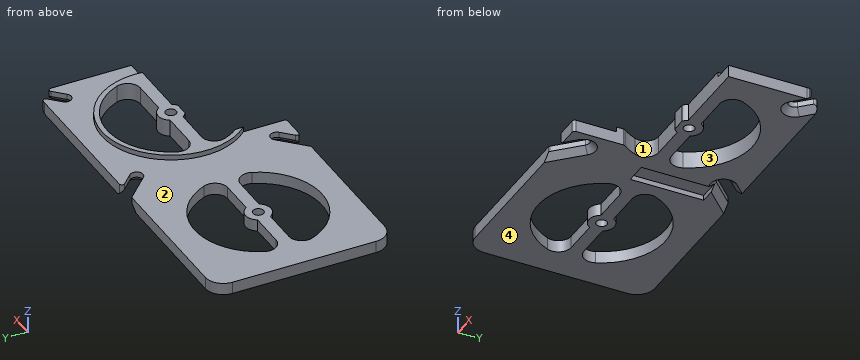
Autodesk Inventor part; units mm, degrees
ref_plane "YZ Plane" through (0, 0, 0) normal (1, 0, 0) x (0, 1, 0)
ref_plane "XZ Plane" through (0, 0, 0) normal (0, 1, 0) x (-1, 0, 0)
ref_plane "XY Plane" through (0, 0, 0) normal (0, 0, 1) x (1, 0, 0)
sketch "Sketch1" plane through (0, 0, 0) normal (0, 0, 1) x (1, 0, 0)
  line L0 (-95.2, -35.2) -> (28.2, -35.2)
  line L1 (35.2, -28.2) -> (35.2, 28.2)
  line L2 (28.2, 35.2) -> (-95.2, 35.2)
  line L3 (-102.2, 28.2) -> (-102.2, -28.2)
  arc A0 (-95.2, 35.2) -> (-102.2, 28.2) centre (-95.2, 28.2) ccw
  arc A1 (35.2, 28.2) -> (28.2, 35.2) centre (28.2, 28.2) ccw
  arc A2 (-102.2, -28.2) -> (-95.2, -35.2) centre (-95.2, -28.2) ccw
  arc A3 (28.2, -35.2) -> (35.2, -28.2) centre (28.2, -28.2) ccw
  line L4 (24.8747, -2.5) -> (24.8747, 2.5) construction
  line L5 (-24.8747, 2.5) -> (-24.8747, -2.5) construction
  line L6 (24.8747, -2.5) -> (-24.8747, 2.5) construction
  line L7 (24.8747, 2.5) -> (-24.8747, -2.5) construction
  arc A4 (-23.1756, -9.375) -> (23.1756, -9.375) centre (0, 0) ccw
  arc A5 (23.1756, 9.375) -> (-23.1756, 9.375) centre (0, 0) ccw
  arc A6 (-18.5405, -2.5) -> (-23.1756, -9.375) centre (-18.5405, -7.5) ccw
  arc A7 (-23.1756, 9.375) -> (-18.5405, 2.5) centre (-18.5405, 7.5) ccw
  arc A8 (23.1756, -9.375) -> (18.5405, -2.5) centre (18.5405, -7.5) ccw
  arc A9 (18.5405, 2.5) -> (23.1756, 9.375) centre (18.5405, 7.5) ccw
  line L8 (-4.3301, 2.5) -> (-18.5405, 2.5)
  line L9 (-18.5405, -2.5) -> (-4.3301, -2.5)
  line L10 (4.3301, -2.5) -> (18.5405, -2.5)
  line L11 (18.5405, 2.5) -> (4.3301, 2.5)
  arc A10 (-4.3301, -2.5) -> (4.3301, -2.5) centre (0, 0) ccw
  arc A11 (4.3301, 2.5) -> (-4.3301, 2.5) centre (0, 0) ccw
  line L12 (-18.5405, 7.5) -> (18.5405, 7.5) construction
  line L13 (18.5405, -7.5) -> (-18.5405, -7.5) construction
  line L14 (0, 0) -> (0, -35.2) construction
  line L15 (0, 0) -> (0, 35.2) construction
  line L16 (0, 0) -> (35.2, 0) construction
  line L17 (-33.5, -35.2) -> (-33.5, 35.2) construction
  arc A12 (-90.1756, -9.375) -> (-43.8244, -9.375) centre (-67, 0) ccw
  arc A13 (-43.8244, 9.375) -> (-90.1756, 9.375) centre (-67, 0) ccw
  arc A14 (-43.8244, -9.375) -> (-48.4595, -2.5) centre (-48.4595, -7.5) ccw
  arc A15 (-48.4595, 2.5) -> (-43.8244, 9.375) centre (-48.4595, 7.5) ccw
  arc A16 (-85.5405, -2.5) -> (-90.1756, -9.375) centre (-85.5405, -7.5) ccw
  arc A17 (-90.1756, 9.375) -> (-85.5405, 2.5) centre (-85.5405, 7.5) ccw
  line L18 (-62.6699, 2.5) -> (-48.4595, 2.5)
  line L19 (-48.4595, -2.5) -> (-62.6699, -2.5)
  line L20 (-71.3301, -2.5) -> (-85.5405, -2.5)
  line L21 (-85.5405, 2.5) -> (-71.3301, 2.5)
  arc A18 (-71.3301, -2.5) -> (-62.6699, -2.5) centre (-67, 0) ccw
  arc A19 (-62.6699, 2.5) -> (-71.3301, 2.5) centre (-67, 0) ccw
  point P0 (0, 0)
  point P1 (0, 0)
  dimension "d63" = 67
  dimension "d1" = 7
  dimension "d3" = 5
  dimension "d4" = 25
  dimension "d5" = 5
  dimension "d7" = 5
  dimension "d59" = 70.4
  dimension "d60" = 137.4
extrude "Extrusion1" add sketch "Sketch1" along normal blind 4.7
sketch "Sketch2" plane through (0, 0, 4.7) normal (0, 0, 1) x (1, 0, 0)
  circle A0 centre (0, 0) radius 27
  arc A1 (23.1756, 9.375) -> (-23.1756, 9.375) centre (0, 0) ccw
  arc A2 (18.5405, 2.5) -> (23.1756, 9.375) centre (18.5405, 7.5) ccw
  line L0 (18.5405, 2.5) -> (4.3301, 2.5)
  arc A3 (4.3301, 2.5) -> (-4.3301, 2.5) centre (0, 0) ccw
  line L1 (-4.3301, 2.5) -> (-18.5405, 2.5)
  arc A4 (-23.1756, 9.375) -> (-18.5405, 2.5) centre (-18.5405, 7.5) ccw
  line L2 (-18.5405, -2.5) -> (-4.3301, -2.5)
  arc A5 (-4.3301, -2.5) -> (4.3301, -2.5) centre (0, 0) ccw
  line L3 (4.3301, -2.5) -> (18.5405, -2.5)
  arc A6 (23.1756, -9.375) -> (18.5405, -2.5) centre (18.5405, -7.5) ccw
  arc A7 (-23.1756, -9.375) -> (23.1756, -9.375) centre (0, 0) ccw
  arc A8 (-18.5405, -2.5) -> (-23.1756, -9.375) centre (-18.5405, -7.5) ccw
  line L4 (28.2, 35.2) -> (-95.2, 35.2)
  arc A9 (-95.2, 35.2) -> (-102.2, 28.2) centre (-95.2, 28.2) ccw
  line L5 (-102.2, 28.2) -> (-102.2, -28.2)
  arc A10 (-102.2, -28.2) -> (-95.2, -35.2) centre (-95.2, -28.2) ccw
  line L6 (-95.2, -35.2) -> (28.2, -35.2)
  arc A11 (28.2, -35.2) -> (35.2, -28.2) centre (28.2, -28.2) ccw
  line L7 (35.2, -28.2) -> (35.2, 28.2)
  arc A12 (35.2, 28.2) -> (28.2, 35.2) centre (28.2, 28.2) ccw
  dimension "d10" = 54
extrude "Extrusion2" add sketch "Sketch2" along normal blind 2 contours A0
sketch "Sketch3" plane through (0, 0, 0) normal (0, 0, -1) x (-1, 0, 0)
  line L0 (-27.5, -27.5) -> (27.5, -27.5) construction
  line L1 (27.5, -27.5) -> (27.5, 27.5) construction
  line L2 (27.5, 27.5) -> (-27.5, 27.5) construction
  line L3 (-27.5, 27.5) -> (-27.5, -27.5) construction
  line L4 (-27.5, -27.5) -> (27.5, 27.5) construction
  line L5 (27.5, -27.5) -> (-27.5, 27.5) construction
  line L6 (-27.5, 27.5) -> (-36.9678, 36.9678) construction
  line L7 (-25.7322, 29.2678) -> (-35.2, 38.7355)
  line L8 (-38.7355, 35.2) -> (-29.2678, 25.7322)
  arc A0 (-29.2678, 25.7322) -> (-25.7322, 29.2678) centre (-27.5, 27.5) ccw
  arc A1 (-35.2, 38.7355) -> (-38.7355, 35.2) centre (-36.9678, 36.9678) ccw
  line L9 (95.2, 35.2) -> (-28.2, 35.2) construction
  arc A2 (-38.7355, -35.2) -> (-35.2, -38.7355) centre (-36.9678, -36.9678) ccw
  line L10 (-29.2678, -25.7322) -> (-38.7355, -35.2)
  line L11 (-35.2, -38.7355) -> (-25.7322, -29.2678)
  arc A3 (-25.7322, -29.2678) -> (-29.2678, -25.7322) centre (-27.5, -27.5) ccw
  arc A4 (35.2, -38.7355) -> (38.7355, -35.2) centre (36.9678, -36.9678) ccw
  line L12 (25.7322, -29.2678) -> (35.2, -38.7355)
  line L13 (38.7355, -35.2) -> (29.2678, -25.7322)
  arc A5 (29.2678, -25.7322) -> (25.7322, -29.2678) centre (27.5, -27.5) ccw
  arc A6 (38.7355, 35.2) -> (35.2, 38.7355) centre (36.9678, 36.9678) ccw
  line L14 (29.2678, 25.7322) -> (38.7355, 35.2)
  line L15 (35.2, 38.7355) -> (25.7322, 29.2678)
  arc A7 (25.7322, 29.2678) -> (29.2678, 25.7322) centre (27.5, 27.5) ccw
  arc A8 (62.6699, -2.5) -> (71.3301, -2.5) centre (67, 0) ccw construction
  line L16 (67, 0) -> (0, 0) construction
  line L17 (134, 0) -> (67, 0) construction
  arc A9 (92.7322, 29.2678) -> (96.2678, 25.7322) centre (94.5, 27.5) ccw
  line L18 (96.2678, 25.7322) -> (105.7355, 35.2)
  arc A10 (105.7355, 35.2) -> (102.2, 38.7355) centre (103.9678, 36.9678) ccw
  line L19 (102.2, 38.7355) -> (92.7322, 29.2678)
  line L20 (28.2645, 35.2) -> (37.7322, 25.7322)
  arc A11 (37.7322, 25.7322) -> (41.2678, 29.2678) centre (39.5, 27.5) ccw
  line L21 (41.2678, 29.2678) -> (31.8, 38.7355)
  arc A12 (31.8, 38.7355) -> (28.2645, 35.2) centre (30.0322, 36.9678) ccw
  line L22 (31.8, -38.7355) -> (41.2678, -29.2678)
  arc A13 (41.2678, -29.2678) -> (37.7322, -25.7322) centre (39.5, -27.5) ccw
  line L23 (37.7322, -25.7322) -> (28.2645, -35.2)
  arc A14 (28.2645, -35.2) -> (31.8, -38.7355) centre (30.0322, -36.9678) ccw
  line L24 (105.7355, -35.2) -> (96.2678, -25.7322)
  arc A15 (96.2678, -25.7322) -> (92.7322, -29.2678) centre (94.5, -27.5) ccw
  line L25 (92.7322, -29.2678) -> (102.2, -38.7355)
  arc A16 (102.2, -38.7355) -> (105.7355, -35.2) centre (103.9678, -36.9678) ccw
  point P0 (-32.2339, 32.2339)
  point P1 (129.6699, -2.5)
  point P2 (138.3301, -2.5)
  dimension "d68" = 55
  dimension "d70" = 5
  dimension "d73" = 360
  dimension "d211" = 67
  dimension "d214" = 67
  dimension "d221" = 360
extrude "Extrusion3" cut sketch "Sketch3" against normal through all contours A0 L8 A1 L7 | L10 A3 L11 A2 | L12 L22 L13 A4 | L12 L23 L13 L22 | L12 A5 L13 L23 | L14 L21 L15 A6 | L14 L20 L15 L21 | L14 A7 L15 L20
chamfer "Chamfer1" distance 2.5 angle 45 12 edges at (28.3939, 31.9294, 0) (25.7322, 25.7322, 0) (31.9294, 28.3939, 0) (-28.6983, 32.2339, 0) (-25.7322, 25.7322, 0) (-34.0017, 30.4661, 0) (-25.7322, -25.7322, 0) (-34.0017, -30.4661, 0) (-28.6983, -32.2339, 0) (25.7322, -25.7322, 0) (28.3939, -31.9294, 0) (31.9294, -28.3939, 0)
fillet "Fillet1" radius 1 8 edges at (34.5911, -31.0555, 3.6) (31.0555, -34.5911, 3.6) (31.0555, 34.5911, 3.6) (34.5911, 31.0555, 3.6) (-31.6645, 35.2, 3.6) (-38.7355, 35.2, 3.6) (-31.6645, -35.2, 3.6) (-38.7355, -35.2, 3.6)
sketch "Sketch7" plane through (0, 0, 0) normal (0, 0, -1) x (-1, 0, 0)
  arc A0 (-4.3301, -2.5) -> (4.3301, -2.5) centre (0, 0) ccw construction
  arc A1 (62.6699, -2.5) -> (71.3301, -2.5) centre (67, 0) ccw
  point P0 (0, 0)
hole "Hole2" at (0, 0, 0) at (-67, 0, 0) direction (0, 0, 1) diameter 4.2 end through all
sketch "Sketch4" plane through (0, 0, 0) normal (0, 0, -1) x (-1, 0, 0)
  line L0 (19.8, -4.2) -> (19.8, -35.2)
  line L1 (19.8, -35.2) -> (-35.2, -35.2)
  line L2 (-35.2, -35.2) -> (-35.2, -4.2)
  line L3 (19.8, -4.2) -> (-35.2, -4.2)
  line L4 (102.2, -35.2) -> (-35.2, -35.2) construction
  line L5 (-35.2, -35.2) -> (-35.2, 35.2) construction
  line L6 (-35.2, 35.2) -> (102.2, 35.2) construction
  line L7 (102.2, 35.2) -> (102.2, -35.2) construction
  line L8 (28.1289, 35.2) -> (42.2711, 35.2) construction
  line L9 (-35.2, 28.1289) -> (-35.2, -28.1289) construction
  line L10 (-28.2, -35.2) -> (28.1289, -35.2) construction
  line L11 (102.2, -28.2) -> (102.2, 28.2) construction
  line L12 (-4.3301, -2.5) -> (-18.5405, -2.5)
  line L13 (-4.3301, -2.5) -> (-35.2, -2.5)
  line L14 (-35.2, -2.5) -> (-35.2, -4.2)
  line L15 (-35.2, -4.2) -> (-4.3301, -4.2)
  line L16 (-4.3301, -4.2) -> (-4.3301, -2.5)
  point P0 (-28.1289, 35.2)
  point P1 (-28.1289, -35.2)
  dimension "d39" = 31
  dimension "d41" = 55
extrude "Extrusion4" cut sketch "Sketch4" against normal through all
fillet "Fillet2" radius 1 2 edges at (-19.8, -15.263, 3.35) (-19.8, -35.2, 2.35)
sketch "Sketch8" plane through (0, 0, 0) normal (0, 0, -1) x (-1, 0, 0)
  line L0 (0, 0) -> (35.5, 0) construction
  line L1 (35.5, 0) -> (71, 0) construction
  line L2 (32.5, 32.5) -> (32.5, -32.5) construction
  line L3 (32.5, -32.5) -> (-32.5, -32.5) construction
  line L4 (-32.5, -32.5) -> (-32.5, 32.5) construction
  line L5 (-32.5, 32.5) -> (32.5, 32.5) construction
  line L6 (99.5, 32.5) -> (99.5, -32.5) construction
  line L7 (99.5, -32.5) -> (34.5, -32.5) construction
  line L8 (34.5, -32.5) -> (34.5, 32.5) construction
  line L9 (34.5, 32.5) -> (99.5, 32.5) construction
  line L10 (96.3694, 32.5) -> (96.3694, 35.2) construction
  line L11 (99.5, 26.6962) -> (102.2, 26.6962) construction
  line L12 (92.7868, -32.5) -> (92.7868, -35.2) construction
  line L13 (102.2, -28.2) -> (102.2, 28.2) construction
  line L14 (42.2711, -35.2) -> (95.2, -35.2) construction
  line L15 (-35.2, -1.5) -> (-35.2, 28.2) construction
  line L16 (-35.2, 21.6184) -> (-32.5, 21.6184) construction
  line L17 (95.2, 35.2) -> (42.2711, 35.2) construction
  line L18 (29.4901, 25.1562) -> (37.9558, 25.1562)
  line L19 (37.9558, 25.1562) -> (37.9558, -3.6366)
  line L20 (37.9558, -3.6366) -> (29.4901, -3.6366)
  line L21 (29.4901, -3.6366) -> (29.4901, 25.1562)
  dimension "d131" = 65
extrude "Extrusion6" cut sketch "Sketch8" against normal blind 2
equation "\"Offset\" = 0.3"
equation "\"d56\" = 0.3"
properties part number "V4 in walldual"
CAD build for the part. Positions are in the model's coordinates, mm. Face numbers are marked on the shaded views. A direction names the side the tool comes from. Coordinates: 2 decimals unless noted, no trailing zeros. Order: outer loops, then holes, each group sorted by start corner. A loop starts at its lowest first (then second) coordinate and runs counter-clockwise, first axis right, second up. Notation, with made-up numbers: M 25.5,67.5 L 66.5,67.5 A18 cw 66.5,93.5 Z; hole C 73,-21 d11. An arc over 180 degrees is marked long. Answer as CSV lines item,"result".
1) Cut at B-B (y = -11). List the corners of the cut face in (x, z).
Verdict:
outline,"M -102.2,0 L -89.45,0 L -89.45,4.7 L -102.2,4.7 Z; M -44.55,0 L -22.45,0 L -22.45,6.7 L -24.66,6.7 L -24.66,4.7 L -44.55,4.7 Z"
2) Drill centre lines: L1, parallel to X at y = 0, z = 3.6; L2, parallel to Y at x = -61, z = 4.25; L3, parallel to Y at x = -51, z = 3.25. Where is each one in solid material? Low to high. Write a range as from..to.
Verdict:
L1,"-102.2..-69.1, -64.9..-2.1, 2.1..35.2"
L2,"-35.2..-24.27, -2.5..2.5, 24.27..35.2"
L3,"-35.2..-19.21, -2.5..2.5, 19.21..35.2"
3) 3-axis set-ups, long thin cutter, end or side, ignore diameter. For the marked faces 3 and 4: which of +Z, -Z, +X, -X, +Y, -Y reach the whole face in a straight line?
Verdict:
face 3,"+Z, -Z"
face 4,"-Z, +X, -X, +Y, -Y"
4) Mould opens along X. For the marked faces 1 and 2 say: released by +X, released by -X, zero draft, split by the parting line, or undercut.
Verdict:
face 1,"undercut"
face 2,"zero draft"
5) Flat gauge pins, fed straight in: P1, Ø5, axis at x = -67, y = 0, coming from the +Z side; P2, Ø3.5, axis at x = 14, z = 2.5, coming from the -Y side; P3, Ø1.5, axis at y = -23, z = 4, coming from the +X side. Where does each tip first touch, or does it go through?
Verdict:
P1,"z = 4.7"
P2,"y = -2.5"
P3,"x = -19.8"
6) Cut at A-A (x = -67). List the corners of the cut face in (y, z), then the cut area to 3 significant figures.
Verdict:
outline,"M -35.2,0 L -25,0 L -25,4.7 L -35.2,4.7 Z; M -5,0 L -2.1,0 L -2.1,4.7 L -5,4.7 Z; M 2.1,0 L 5,0 L 5,4.7 L 2.1,4.7 Z; M 25,0 L 35.2,0 L 35.2,4.7 L 25,4.7 Z"
area,"123 mm2"
